Autodesk Inventor part; units mm, degrees
ref_plane "YZ Plane" through (0, 0, 0) normal (1, 0, 0) x (0, 1, 0)
ref_plane "XZ Plane" through (0, 0, 0) normal (0, 1, 0) x (-1, 0, 0)
ref_plane "XY Plane" through (0, 0, 0) normal (0, 0, 1) x (1, 0, 0)
sketch "Эскиз1" plane through (0, 0, 0) normal (0, 0, 1) x (1, 0, 0)
  line L0 (0, 0) -> (24, 0)
  line L1 (24, 0) -> (24, 7)
  line L2 (24, 7) -> (0, 7)
  line L3 (0, 7) -> (0, 0)
  line L4 (0, 1) -> (24, 1)
  line L5 (2, 7) -> (2, 0)
  line L6 (22, 7) -> (22, 0)
  point P0 (0, 3.5)
  point P1 (12, 0)
  point P2 (2, 1)
  point P3 (22, 1)
  dimension "d0" = 24
  dimension "d1" = 7
  dimension "d2" = 2
  dimension "d3" = 2
  dimension "d4" = 1
extrude "Выдавливание1" add sketch "Эскиз1" along normal blind 397 contours L3 L4 L5 L0 | L5 L4 L6 L0 | L3 L2 L5 L4 | L6 L4 L1 L0 | L6 L2 L1 L4
sketch "Эскиз3" plane through (0, 0, 0) normal (0, -1, 0) x (1, 0, 0)
  line L0 (12.0033, 0) -> (12, 397)
  line L1 (22, 397) -> (2, 397)
  line L2 (24, 0) -> (24, 397)
  circle A0 centre (12.0005, 336) radius 2.25
  line L3 (12.0002, 366.75) -> (12.0003, 357.25) construction
  line L4 (9.7503, 364.5) -> (9.7503, 359.5)
  line L5 (14.2503, 359.5) -> (14.2503, 364.5)
  arc A1 (14.2503, 364.5) -> (9.7503, 364.5) centre (12.0003, 364.5) ccw
  arc A2 (9.7503, 359.5) -> (14.2503, 359.5) centre (12.0003, 359.5) ccw
  line L6 (16.7506, 346) -> (7.2506, 346) construction
  line L7 (14.5006, 348.25) -> (9.5006, 348.25)
  line L8 (9.5007, 343.75) -> (14.5007, 343.75)
  arc A3 (14.5007, 343.75) -> (14.5006, 348.25) centre (14.5006, 346) ccw
  arc A4 (9.5006, 348.25) -> (9.5007, 343.75) centre (9.5006, 346) ccw
  circle A5 centre (12.0013, 214) radius 2.25
  line L9 (12.001, 244.75) -> (12.0011, 235.25) construction
  line L10 (9.751, 242.5) -> (9.7511, 237.5)
  line L11 (14.2511, 237.5) -> (14.251, 242.5)
  arc A6 (14.251, 242.5) -> (9.751, 242.5) centre (12.001, 242.5) ccw
  arc A7 (9.7511, 237.5) -> (14.2511, 237.5) centre (12.0011, 237.5) ccw
  arc A8 (9.5014, 226.25) -> (9.5014, 221.75) centre (9.5014, 224) ccw
  line L12 (9.5014, 221.75) -> (14.5014, 221.75)
  line L13 (14.5014, 226.25) -> (9.5014, 226.25)
  line L14 (16.7514, 224) -> (7.2514, 224) construction
  arc A9 (14.5014, 221.75) -> (14.5014, 226.25) centre (14.5014, 224) ccw
  line L15 (9.5031, 93.75) -> (14.5031, 93.75)
  line L16 (16.7531, 96) -> (7.2531, 96) construction
  arc A10 (9.5031, 98.25) -> (9.5031, 93.75) centre (9.5031, 96) ccw
  line L17 (14.5031, 98.25) -> (9.5031, 98.25)
  arc A11 (14.5031, 93.75) -> (14.5031, 98.25) centre (14.5031, 96) ccw
  circle A12 centre (12.003, 86) radius 2.25
  arc A13 (9.7528, 109.5) -> (14.2528, 109.5) centre (12.0028, 109.5) ccw
  line L18 (14.2528, 109.5) -> (14.2528, 114.5)
  line L19 (9.7528, 114.5) -> (9.7528, 109.5)
  arc A14 (14.2528, 114.5) -> (9.7528, 114.5) centre (12.0028, 114.5) ccw
  line L20 (12.0027, 116.75) -> (12.0028, 107.25) construction
  circle A15 centre (12.0023, 123) radius 2.5
  point P0 (12.0003, 362)
  point P1 (12.0006, 346)
  point P2 (12.001, 240)
  point P3 (12.0014, 224)
  point P4 (12.0031, 96)
  point P5 (12.0028, 112)
  dimension "d47" = 4.5
  dimension "d49" = 9.5
  dimension "d50" = 4.5
  dimension "d51" = 9.5
  dimension "d52" = 4.5
  dimension "d53" = 10
  dimension "d54" = 16
  dimension "d55" = 70
  dimension "d56" = 4.5
  dimension "d57" = 9.5
  dimension "d58" = 4.5
  dimension "d59" = 9.5
  dimension "d60" = 4.5
  dimension "d61" = 10
  dimension "d62" = 16
  dimension "d63" = 138
  dimension "d64" = 4.5
  dimension "d65" = 9.5
  dimension "d66" = 4.5
  dimension "d67" = 9.5
  dimension "d68" = 4.5
  dimension "d69" = 10
  dimension "d70" = 16
  dimension "d71" = 138
  dimension "d72" = 5
extrude "Выдавливание2" cut sketch "Эскиз3" against normal blind 10
sketch "Эскиз4" plane through (0, 0, 0) normal (0, 0, -1) x (-1, 0, 0)
  line L0 (-2, 7) -> (0, 7)
  line L1 (-2, 1) -> (-2, 7)
  line L2 (-22, 1) -> (-2, 1)
  line L3 (-22, 7) -> (-22, 1)
  line L4 (-24, 7) -> (-22, 7)
  line L5 (-24, 0) -> (-24, 7)
  line L6 (0, 0) -> (-24, 0)
  line L7 (0, 7) -> (0, 0)
  line L8 (-12, 9) -> (-20, 9)
  line L9 (-20, 9) -> (-20, 0)
  line L10 (-12, 9) -> (-4, 9)
  line L11 (-4, 9) -> (-4, 0)
  point P0 (-20, 1)
  point P1 (-4, 1)
extrude "Выдавливание3" add sketch "Эскиз4" against normal blind 1.5 contours L2 L9 L8 L10 L11
sketch "Эскиз5" plane through (0, 0, 0) normal (0, 0, -1) x (-1, 0, 0)
  line L0 (0, 0) -> (-24, 0)
  line L1 (-24, 7) -> (-21.5, 7)
  line L2 (-21.5, 7) -> (-21.5, 0)
  line L3 (-21.5, 0) -> (-24, 0)
  line L4 (-24, 0) -> (-24, 7)
  line L5 (0, 7) -> (-2.5, 7)
  line L6 (-2.5, 7) -> (-2.5, 0)
  line L7 (-2.5, 0) -> (0, 0)
  line L8 (0, 0) -> (0, 7)
  line L9 (-21.5, 7) -> (-19.5, 7)
  line L10 (-19.5, 7) -> (-19.5, 0)
  line L11 (-19.5, 0) -> (-21.5, 0)
  line L12 (-21.5, 0) -> (-21.5, 7)
  line L13 (-2.5, 7) -> (-4.5, 7)
  line L14 (-4.5, 7) -> (-4.5, 0)
  line L15 (-4.5, 0) -> (-2.5, 0)
  line L16 (-2.5, 0) -> (-2.5, 7)
  line L17 (-19.5, 0) -> (-17.5, 0)
  line L18 (-4.5, 0) -> (-6.5, 0)
  line L19 (-20, 9) -> (-4, 9)
  line L20 (-17.5, 0) -> (-6.5, 0)
  line L21 (-6.5, 0) -> (-6.5, 9)
  line L22 (-6.5, 9) -> (-17.5, 9)
  line L23 (-17.5, 9) -> (-17.5, 0)
  line L24 (-17.5, 7) -> (-21, 7)
  line L25 (-21, 7) -> (-21, 9)
  line L26 (-21, 9) -> (-17.5, 9)
  line L27 (-17.5, 9) -> (-17.5, 7)
  line L28 (-6.5, 7) -> (-4, 7)
  line L29 (-4, 7) -> (-4, 9)
  line L30 (-4, 9) -> (-6.5, 9)
  line L31 (-6.5, 9) -> (-6.5, 7)
  dimension "d36" = 2.5
  dimension "d37" = 2.5
  dimension "d38" = 2
  dimension "d39" = 2
  dimension "d40" = 2
  dimension "d41" = 2
extrude "Выдавливание4" cut sketch "Эскиз5" against normal through all contours L0 L6 L5 L8 | L0 L21 L28 L14 | L28 L21 L19 L29 L13 | L0 L10 L24 L23 | L24 L9 L25 L26 L19 L23 | L0 L4 L1 L2
sketch "Эскиз6" plane through (0, 0, 0) normal (0, 0, -1) x (-1, 0, 0)
  line L0 (-19.5, 0) -> (-21.5, 0)
  line L1 (-19.5, 0) -> (-19.5, 7)
  line L2 (-21.5, 0) -> (-19.5, 0)
  line L3 (-19.5, 0) -> (-19.5, 7)
  line L4 (-19.5, 7) -> (-21.5, 7)
  line L5 (-21.5, 7) -> (-21.5, 0)
  line L6 (-4.5, 1) -> (-4.5, 7)
  line L7 (-2.5, 0) -> (-4.5, 0)
  line L8 (-4.5, 7) -> (-2.5, 7)
  line L9 (-2.5, 7) -> (-2.5, 0)
  line L10 (-2.5, 0) -> (-4.5, 0)
  line L11 (-4.5, 0) -> (-4.5, 7)
  line L12 (-21.5, 1) -> (-2.5, 1)
  line L13 (-2.5, 1) -> (-2.5, 0)
  line L14 (-2.5, 0) -> (-21.5, 0)
  line L15 (-21.5, 0) -> (-21.5, 1)
  line L16 (-6.5, 0) -> (-6.5, 9)
  line L17 (-6.5, 1) -> (-6.5, 0)
  line L18 (-17.5, 1) -> (-6.5, 1)
  line L19 (-17.5, 9) -> (-17.5, 0)
  line L20 (-17.5, 1) -> (-17.5, 0)
  point P0 (0, 0)
  point P1 (-19.5, 1)
extrude "Выдавливание5" add sketch "Эскиз6" against normal up to surface (397 mm away) contours L1 L12 L19 L14 | L12 L5 L4 L1 | L16 L12 L11 L14 | L6 L8 L9 L12
sketch "Эскиз7" plane through (2.5, 0, 0) normal (0, -1, 0) x (1, 0, 0)
  line L0 (0, 397) -> (19, 397)
  line L1 (9.5, 397) -> (2.5, 397)
  line L2 (9.5, 397) -> (16.5, 397)
  line L3 (16.5, 397) -> (16.5, 387)
  line L4 (16.5, 387) -> (2.5, 387)
  line L5 (2.5, 387) -> (2.5, 397)
  point P0 (-2.5, 0)
  dimension "d73" = 7
  dimension "d74" = 7
  dimension "d75" = 10
extrude "Выдавливание6" cut sketch "Эскиз7" against normal blind 10
fillet "Сопряжение1" radius 1 4 edges at (5, 0.5, 387) (19, 0.5, 387) (19, 0.5, 397) (5, 0.5, 397)
sketch "Эскиз8" plane through (0, 0, 0) normal (0, 0, -1) x (-1, 0, 0)
  line L0 (-6.5, 9) -> (-17.5, 9)
  line L1 (-17.5, 9) -> (-17.5, 1)
  line L2 (-6.5, 9) -> (-17.5, 9)
  line L3 (-17.5, 9) -> (-17.5, 6)
  line L4 (-17.5, 6) -> (-6.5, 6)
  line L5 (-6.5, 6) -> (-6.5, 9)
  point P0 (0, 0)
extrude "Выдавливание7" cut sketch "Эскиз8" against normal blind 10
sketch "Эскиз9" plane through (0, 0, 1.5) normal (0, 0, 1) x (1, 0, 0)
  line L0 (17.5, 6) -> (6.5, 6)
  line L1 (6.5, 6) -> (6.5, 1)
  line L2 (17.5, 1) -> (6.5, 1)
  line L3 (17.5, 1) -> (17.5, 6)
  point P0 (0, 0)
extrude "Выдавливание8" add sketch "Эскиз9" along normal blind 50
sketch "Эскиз10" plane through (0, 0, 0) normal (0, 0, -1) x (-1, 0, 0)
  line L0 (-30, 24) -> (32, 24)
  line L1 (32, 24) -> (32, -21)
  line L2 (32, -21) -> (-30, -21)
  line L3 (-30, -21) -> (-30, 24)
  point P0 (0, 0)
extrude "Выдавливание9" cut sketch "Эскиз10" against normal blind 50
equation "\"d31\" = d61"
equation "\"d76\" = d61"
equation "\"d79\" = d61"
properties part number "3 часть направляшки 35"
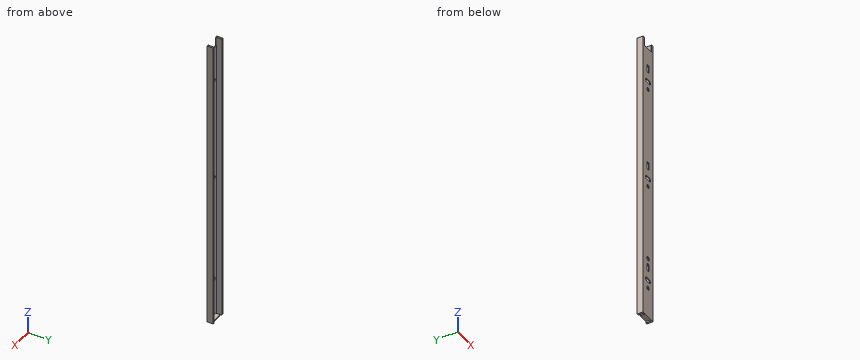
The listing builds one solid part. Answer for the finished solid, in the listing's coordinates (mm). Give positions to 0.01 mm unless a question says otherwise; leave off trailing zeros. Write each loop counter-clockwise with the first axis right and the second up, starting at its lowest first coordinate (ties: lowest second). Pieces come first, ordered by that corner, then holes. Notation, with made-up numbers: (13.5, 44) -> (26.5, 44) arc R17 cw to (26.5, 65) -> close; hole circle Ø5 at (87.5, 40). An arc over 180 degrees is marked (long way). Use a Markdown table: item, result.
(1) Section B-B, the plane z = 302 is taken. Determine the outline of the cut face in (x, y).
Return value:
| item | result |
|---|---|
| outline | (2.5, 0) -> (21.5, 0) -> (21.5, 7) -> (19.5, 7) -> (19.5, 1) -> (4.5, 1) -> (4.5, 7) -> (2.5, 7) -> close |
(2) Section A-A, the plane y = 3.5 is taken. Determine the outline of the cut face in (x, z), then the cut area to 3 significant figures.
Return value:
| item | result |
|---|---|
| outline | (2.5, 50) -> (4.5, 50) -> (4.5, 396.87) arc R1 ccw to (4, 397) -> (2.5, 397) -> close; (6.5, 50) -> (17.5, 50) -> (17.5, 51.5) -> (6.5, 51.5) -> close; (19.5, 50) -> (21.5, 50) -> (21.5, 397) -> (20, 397) arc R1 ccw to (19.5, 396.87) -> close |
| area | 1,400 mm2 |
(3) Flat-ended cylindrical pins translate along their axes: P1, Ø5, axis at x = 12, z = 336, coming from the +Y side; P2, Ø1.1, axis at x = 13, y = 0.5, coming from the +Z side; P3, Ø1.6, axis at x = 11.5, z = 51, coming from the +Y side. Find the tip coordinate at first contact, or state that the pin passes through.
Return value:
| item | result |
|---|---|
| P1 | y = 1 |
| P2 | z = 387 |
| P3 | y = 6 |
(4) Find the intervals of material crossed by probe 1 along X at (y, z) = (6.75, 106); probe 2 along X at (y, z) = (0.35, 336); probe 3 along Y at (x, z) = (8.75, 229.5), in increasing order. Write a range as from..to.
Return value:
| item | result |
|---|---|
| probe 1 | 2.5..4.5, 19.5..21.5 |
| probe 2 | 2.5..9.75, 14.25..21.5 |
| probe 3 | 0..1 |
